from build123d import *

# Parameters (mm, degrees)
F1_DEPTH = 76.2
F3_DEPTH = 25.4


with BuildPart() as f1:
    # F0 (on Front) → F1 (new body)
    with BuildSketch(Plane.XZ):
        Polygon((-38.1, -12.7), (38.1, -12.7), (38.1, 12.7), (25.4, 12.7), (25.4, 7.089494), (12.7, 7.089494), (12.7, 12.7), (-38.1, 12.7), align=None)
    extrude(amount=F1_DEPTH)

    # F2 (on face) → F3 (cut)
    with BuildSketch(Plane.XY.offset(12.7)):
        with BuildLine():
            ThreePointArc((-3.175, -25.4), (-5.964808, -18.664808), (-12.7, -15.875))
            Line((-12.7, -15.875), (-12.7, -25.4))
            Line((-12.7, -25.4), (-22.225, -25.4))
            ThreePointArc((-22.225, -25.4), (-12.7, -34.925), (-3.175, -25.4))
        make_face()
        with BuildLine():
            Line((-12.7, -25.4), (-12.7, -15.875))
            ThreePointArc((-12.7, -15.875), (-19.435192, -18.664808), (-22.225, -25.4))
            Line((-22.225, -25.4), (-12.7, -25.4))
        make_face()
    extrude(amount=-F3_DEPTH, mode=Mode.SUBTRACT)


solid = f1.part
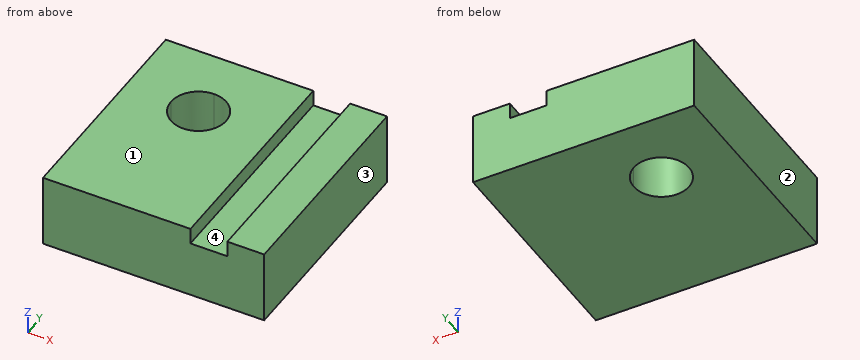
Verification items for the finished model (mm, model axes). Face numbers are marked on the shaded views. Give positions to 0.01 mm unless a question says otherwise; leave off trailing zeros. Loops run counter-clockwise (first coordinate to the right, second up) from the corner with the lowest first, then second, coordinate; pieces in that order, holes last.
1. Cross-section at D-D on z = 4. Record the cut outline in (x, y) (3 decimals), and give its area (3 significant figures).
Derived:
outline: (-38.1, -76.2) - (38.1, -76.2) - (38.1, 0) - (-38.1, 0) - close; hole circle Ø19.05 at (-12.7, -25.4)
area: 5,520 mm2
2. Release check for a two-part mould opening along X. For the marked faces 1, 2, 3 and 4 record: +X half, -X half, draft (parallel to the pull), parting line (faces both ways), or undercut.
Derived:
face 1: draft
face 2: -X half
face 3: +X half
face 4: undercut
3. Go/stop test with a flat-tipped pin: P1, Ø10, axis at x = 18, y = -43.5, coming from the +Z side. Record where the tip stops, or that it passes through.
Derived:
P1: stops at z = 7.09
4. Cross-section at C-C on y = -23. Record the cut outline in (x, z), and give its area (3 significant figures).
Derived:
outline: (-38.1, -12.7) - (-21.92, -12.7) - (-21.92, 12.7) - (-38.1, 12.7) - close; (-3.48, -12.7) - (38.1, -12.7) - (38.1, 12.7) - (25.4, 12.7) - (25.4, 7.09) - (12.7, 7.09) - (12.7, 12.7) - (-3.48, 12.7) - close
area: 1,400 mm2
5. Cross-section at A-A on z = 11.25. Record the cut outline in (x, y) (3 decimals).
Derived:
outline: (-38.1, -76.2) - (12.7, -76.2) - (12.7, 0) - (-38.1, 0) - close; (25.4, -76.2) - (38.1, -76.2) - (38.1, 0) - (25.4, 0) - close; hole circle Ø19.05 at (-12.7, -25.4)
6. Material ranges on probe 1 along X at (y, z) = (-25.5, 1.25); probe 2 along Z at (x, y) = (20, -41); probe 3 along Y at (x, z) = (-21.5, -6.25), recorded low to high.
Derived:
probe 1: x = -38.1 to -22.22, -3.18 to 38.1
probe 2: z = -12.7 to 7.09
probe 3: y = -76.2 to -29.04, -21.76 to 0
7. Cross-section at B-B on y = -46. Record the cut outline in (x, z), and give its area (3 significant figures).
Derived:
outline: (-38.1, -12.7) - (38.1, -12.7) - (38.1, 12.7) - (25.4, 12.7) - (25.4, 7.09) - (12.7, 7.09) - (12.7, 12.7) - (-38.1, 12.7) - close
area: 1,860 mm2
